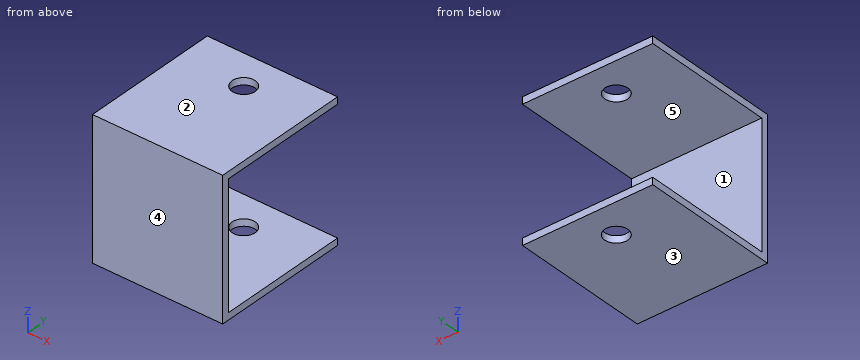
from build123d import *

# Parameters (mm, degrees)
SKETCH1_W               = 35.71875
SKETCH1_H               = 38.1
BOSS_EXTRUDE1_DEPTH     = 38.1
SKETCH2_W               = 34.29
SKETCH2_H               = 36.195
CUT_EXTRUDE1_DEPTH      = 65.645565212
CUT_EXTRUDE2_DEPTH      = 64.541459903
CUT_EXTRUDE2_DEPTH_BACK = 64.541459903
SKETCH3_R               = 3.175


with BuildPart() as part:
    # Sketch1 → Boss-Extrude1 (new body)
    with BuildSketch(Plane.XY):
        with Locations((-17.859375, 19.05)):
            Rectangle(SKETCH1_W, SKETCH1_H)
    extrude(amount=BOSS_EXTRUDE1_DEPTH)

    # Sketch2 → Cut-Extrude1 (cut, through all)
    with BuildSketch(Plane.ZY.offset(35.71875)):
        with Locations((19.05, 20.0025)):
            Rectangle(SKETCH2_W, SKETCH2_H)
    extrude(amount=-CUT_EXTRUDE1_DEPTH, mode=Mode.SUBTRACT)

    # Sketch3 → Cut-Extrude2 (cut, two sides: drawn at the far end of the back side and taken through both)
    with BuildSketch(Plane(origin=(0, 0, 36.195), x_dir=(-1, 0, 0), z_dir=(0, 0, -1)).offset(-CUT_EXTRUDE2_DEPTH_BACK)):
        with Locations(Location((17.859375, 28.575, 0), (0, 0, 90))):
            Circle(SKETCH3_R)
    extrude(amount=CUT_EXTRUDE2_DEPTH + CUT_EXTRUDE2_DEPTH_BACK, mode=Mode.SUBTRACT)


solid = part.part
CAD build for the part. Positions are in the model's coordinates, mm. Face numbers are marked on the shaded views. A direction names the side the tool comes from. Round coordinates to 2 decimals unless told otherwise and drop trailing zeros. Write each loop counter-clockwise with the first axis right and the second up, starting at its lowest first coordinate (ties: lowest second). Pieces come first, ordered by that corner, then holes. Notation, with made-up numbers: (-7.75, -27.5) -> (21.25, -27.5) arc R25 ccw to (21.25, -5.5) -> close; hole circle Ø5 at (20, -11). An arc over 180 degrees is marked (long way). Answer as a JSON object with one key per item and string values.
(1) Band-saw the part on D-D, the plane z = 30. List the corners of the cut face in (x, y) (3 decimals).
Reported:
{"outline": "(-35.719, 0) -> (0, 0) -> (0, 1.905) -> (-35.719, 1.905) -> close"}
(2) Probe probe 1 along Z at (x, y) = (-30, 24.5) (3 decimals); probe 2 along Y at (x, z) = (-19.5, 34.5) (3 decimals). List the from-to ranges inside material, lowest first. Write a range as [from, to].
Reported:
{"probe 1": "z = [0, 1.905], [36.195, 38.1]", "probe 2": "y = [0, 1.905]"}
(3) Pin check, flat tips, straight feed: P1, Ø2, axis at x = -16.5, y = 30, coming from the +Z side; P2, Ø2, axis at x = -30, z = 28.5, coming from the +Y side (3 decimals). Stop position of each tip, or through.
Reported:
{"P1": "passes through", "P2": "stops at y = 1.905"}
(4) Band-saw the part on C-C, the plane y = 30.5. List the corners of the cut face in (x, z) (1 decimal), then the cut area to 3 significant figures.
Reported:
{"outline": "(-35.7, 0) -> (-20.4, 0) -> (-20.4, 1.9) -> (-35.7, 1.9) -> close; (-35.7, 36.2) -> (-20.4, 36.2) -> (-20.4, 38.1) -> (-35.7, 38.1) -> close; (-15.3, 0) -> (0, 0) -> (0, 1.9) -> (-15.3, 1.9) -> close; (-15.3, 36.2) -> (0, 36.2) -> (0, 38.1) -> (-15.3, 38.1) -> close", "area": "117 mm^2"}
(5) Which spindle directions (+Z, -Z, +X, -X, +Y, -Y) get a long thin tool onto all of the face, cutting with end or side? Do the marked faces 4 and 5. Say none if no direction does.
Reported:
{"face 4": "+Z, -Z, +X, -X, -Y", "face 5": "+X, -X, +Y"}
(6) Band-saw the part on A-A, the plane y = 20. List the corners of the cut face in (x, z) (3 decimals), then the cut area to 3 significant figures.
Reported:
{"outline": "(-35.719, 0) -> (0, 0) -> (0, 1.905) -> (-35.719, 1.905) -> close; (-35.719, 36.195) -> (0, 36.195) -> (0, 38.1) -> (-35.719, 38.1) -> close", "area": "136 mm^2"}
(7) Band-saw the part on B-B, the plane x = -31.5. List the corners of the cut face in (y, z) (3 decimals), then the cut area to 3 significant figures.
Reported:
{"outline": "(0, 0) -> (38.1, 0) -> (38.1, 1.905) -> (1.905, 1.905) -> (1.905, 36.195) -> (38.1, 36.195) -> (38.1, 38.1) -> (0, 38.1) -> close", "area": "210 mm^2"}
(8) Two-plate mould, pull along Z, no slides. Class the marked faces 1, 2 and 3: +Z half, -Z half, draft (parallel to the pull), parting line (faces both ways), or undercut.
Reported:
{"face 1": "undercut", "face 2": "+Z half", "face 3": "-Z half"}
